For this review, take the finished solid that the model builds, in its own axes (mm). A direction names the side the tool comes from. Coordinates: 2 decimals unless noted, no trailing zeros. Write each loop counter-clockwise with the first axis right and the second up, starting at its lowest first coordinate (ties: lowest second). Pieces come first, ordered by that corner, then holes. Notation, with made-up numbers: M 75,34.5 L 117,34.5 A13 ccw 117,57.5 Z; hole C -24.75,-22 d11. An arc over 180 degrees is marked long. One line per question, with ' | ' between items.
Autodesk Fusion 360 part; units mm, degrees
sketch "Sketch1" plane through (0, 0, 0) normal (0, 0, 1) x (1, 0, 0)
  line L0 (0, 0) -> (-100, 0) construction
  line L1 (0, 0) -> (100, 0) construction
  line L2 (0, 0) -> (0, 100) construction
  line L3 (0, 0) -> (0, -100) construction
  circle A0 centre (0, 24.5) radius 24.5 construction
  line L4 (30.5, 0) -> (30.5, -100) construction
  line L5 (30.5, 0) -> (30.5, 100) construction
  line L6 (-30.5, 0) -> (-30.5, -100) construction
  line L7 (-30.5, 0) -> (-30.5, 100) construction
  line L8 (0, 49) -> (0, 54) construction
  line L9 (25.5, 0) -> (25.5, 23.5)
  line L10 (-25.5, 0) -> (-25.5, 23.5)
  line L11 (0, 49) -> (0, 49)
  line L12 (0, 49) -> (0, 49)
  arc A1 (0, 49) -> (-25.5, 23.5) centre (0, 23.5) ccw
  arc A2 (25.5, 23.5) -> (0, 49) centre (0, 23.5) ccw
  line L13 (-25.5, 0) -> (-25.5, -20)
  line L14 (25.5, 0) -> (25.5, -20)
  dimension "d5" = 49
  dimension "d6" = 30.5
  dimension "d7" = 30.5
  dimension "d11" = 25.5
  dimension "d12" = 25.5
  dimension "d13" = 20
  dimension "d14" = 20
sketch "Sketch2" plane through (0, 0, 0) normal (1, 0, 0) x (0, 0, -1)
  circle A0 centre (0, 54) radius 5
  point P0 (0, 49)
  dimension "d15" = 10
sweep "Sweep1" add profiles "Sketch2" path "Sketch1" along L14 L9 A2 A1 L10 L13 section 1
chamfer "Chamfer1" distance 1.5 angle 45 2 edges at (-32.3081, -20, 4.6616) (28.6919, -20, 4.6616)
thread "Thread1"
thread "Thread2"
1) We need section B-B on y = 18. State the section outline as (x, z) points.
Responses:
outline: C -30.5,0 d10; C 30.5,0 d10
2) We need section A-A on z = 0. State the section outline as (x, y) points.
Responses:
outline: M -35.5,-18.5 L -34,-20 L -27,-20 L -25.5,-18.5 L -25.5,23.5 A25.5 cw 25.5,23.5 L 25.5,-18.5 L 27,-20 L 34,-20 L 35.5,-18.5 L 35.5,23.5 A35.5 ccw -35.5,23.5 Z
3) Machinability: for faces 3 (the flat face through (31, -20, 0)), 4 (the cylindrical face through (-25.62, 2.79, 1.08)), which of the approach directions +Z, -Z, +X, -X, +Y, -Y give a long, thin tool a straight path to every point of the face, cutting with its end or side? Answer none if there is none.
Responses:
face 3: +Z, -Z, +X, -X, -Y | face 4: -Y
4) To check wall thickness, follow line 1 along X through (y, z) = (-11.5, 0.25); line 2 along X through (y, z) = (-0.5, 2.25); line 3 along Y through (x, z) = (6, -0.5). State the ranges of each line that lie inside material, in increasing order. Write a range as [from, to].
Responses:
line 1: [-35.49, -25.51], [25.51, 35.49] | line 2: [-34.97, -26.03], [26.03, 34.97] | line 3: [48.31, 58.46]
5) Insertion check: pin 1 Ø1 at (x, z) = (11.5, -4) entering from +Y; pin 2 Ø12 at (x, y) = (20, 16) entering from +Z; pin 3 Ø1 at (y, z) = (30, 1) entering from +X; pin 4 Ø1 at (x, y) = (23.5, -9.5) entering from +Z. Each pin has a flat end and moves straight along its axis. Give the tip position at first contact, or say it passes through.
Responses:
pin 1: y = 55.6 | pin 2: z = 2.18 | pin 3: x = 34.92 | pin 4: through
6) The part is to be moulded in two halves that separate along X. For faces 1 (the flat face through (-30, -20, 0)), 2 (the cylindrical face through (25.62, 2.21, 1.08)), say which applies: +X half, -X half, draft (parallel to the pull), parting line (faces both ways), or undercut.
Responses:
face 1: draft | face 2: undercut
